Check sheet for the drawn part. Datum: minimum x, y, z corner. Units: mm. Coordinates: 2 decimals unless noted, no trailing zeros. Order: outer loops, then holes, each group sorted by start corner. A loop starts at its lowest first (then second) coordinate and runs counter-clockwise, first axis right, second up. Notation, with made-up numbers: (22, 41) - (38, 41) arc R23 ccw to (38, 62) - close; hole circle Ø2 at (-21.5, 0.25). An arc over 180 degrees is marked (long way). One line per item, written item: value. Start each with the question number.
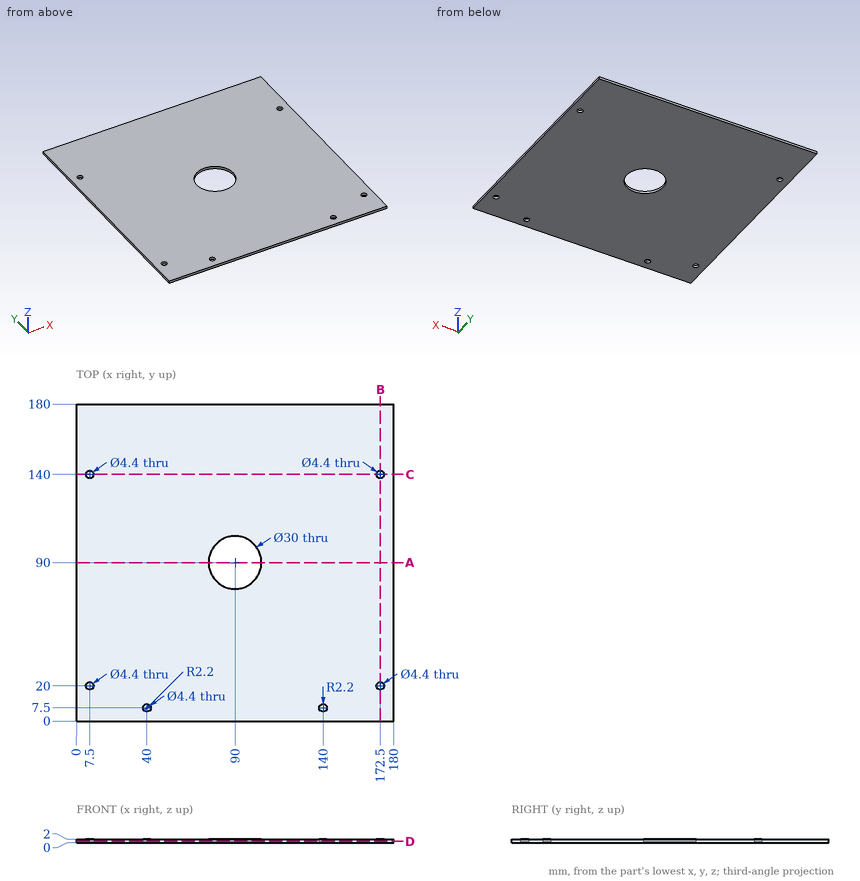
Q1. Cross-section at C-C, the plane y = 140. Enter the section's corners in (x, z), and give its area (3 significant figures).
Q2. Cross-section at A-A, the plane y = 90. Enter the section's corners in (x, z), and give its area (3 significant figures).
Q3. Cross-section at D-D, the plane z = 0.7. Enter the section's corners in (x, y).
Q4. Material ranges on probe 1 along Y at (x, z) = (172.5, 0.55); probe 2 along X at (y, z) = (19, 0.1); probe 3 along X at (y, z) = (140, 0.5), recorded low to high.
Q5. Cross-section at B-B, the plane x = 172.5. Enter the section's corners in (y, z).
Check result:
1. outline: (0, 0) - (5.3, 0) - (5.3, 2) - (0, 2) - close; (9.7, 0) - (170.3, 0) - (170.3, 2) - (9.7, 2) - close; (174.7, 0) - (180, 0) - (180, 2) - (174.7, 2) - close
1. area: 342 mm2
2. outline: (0, 0) - (75, 0) - (75, 2) - (0, 2) - close; (105, 0) - (180, 0) - (180, 2) - (105, 2) - close
2. area: 300 mm2
3. outline: (0, 0) - (180, 0) - (180, 180) - (0, 180) - close; hole circle Ø4.4 at (7.5, 20); hole circle Ø4.4 at (7.5, 140); hole circle Ø4.4 at (40, 7.5); hole circle Ø30 at (90, 90); hole circle Ø4.4 at (140, 7.5); hole circle Ø4.4 at (172.5, 20); hole circle Ø4.4 at (172.5, 140)
4. probe 1: y = 0 to 17.8, 22.2 to 137.8, 142.2 to 180
4. probe 2: x = 0 to 5.54, 9.46 to 170.54, 174.46 to 180
4. probe 3: x = 0 to 5.3, 9.7 to 170.3, 174.7 to 180
5. outline: (0, 0) - (17.8, 0) - (17.8, 2) - (0, 2) - close; (22.2, 0) - (137.8, 0) - (137.8, 2) - (22.2, 2) - close; (142.2, 0) - (180, 0) - (180, 2) - (142.2, 2) - close
